The model under review builds one solid part; all positions refer to its coordinate system, in mm. Face numbers are marked on the shaded views. A direction names the side the tool comes from. Give positions to 0.01 mm unless a question says otherwise; leave off trailing zeros. Loops run counter-clockwise (first coordinate to the right, second up) from the corner with the lowest first, then second, coordinate; pieces in that order, holes last. Notation, with made-up numbers: M 76.5,43.5 L 130.5,43.5 A22 ccw 130.5,80.5 Z; hole C -12,24.25 d6. An arc over 180 degrees is marked long. Put each result on its own line as item: value. Start each with the question number.
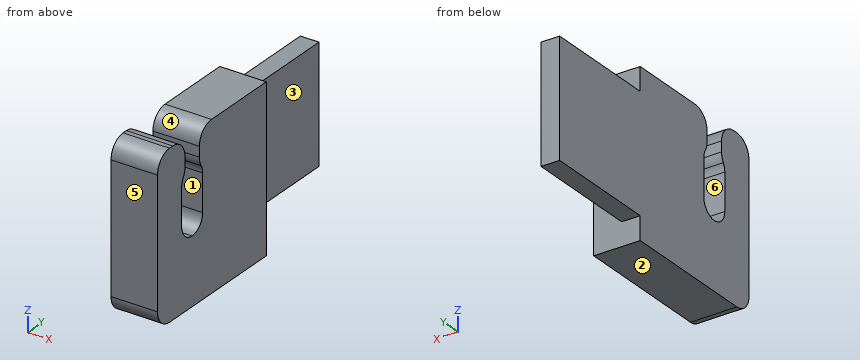
```python
from build123d import *

# Parameters (mm, degrees)
SKETCH1_W           = 10
SKETCH1_H           = 10
BOSS_EXTRUDE1_DEPTH = 1.6
BOSS_EXTRUDE2_DEPTH = 10
SKETCH3_W           = 4
SKETCH3_H           = 2
BOSS_EXTRUDE3_DEPTH = 2
SKETCH4_W           = 4
SKETCH4_H           = 2
BOSS_EXTRUDE4_DEPTH = 2
BOSS_EXTRUDE5_DEPTH = 4
FILLET1_R           = 1.5


with BuildPart() as part:
    # Sketch1 → Boss-Extrude1 (new body)
    with BuildSketch(Plane(origin=(0, 0, 0), x_dir=(0, 0, -1), z_dir=(1, 0, 0))):
        with Locations((5, -5)):
            Rectangle(SKETCH1_W, SKETCH1_H)
    extrude(amount=BOSS_EXTRUDE1_DEPTH)

    # Sketch2 → Boss-Extrude2 (add)
    with BuildSketch(Plane.XY):
        Polygon((1.2, -12), (0, -12), (0, -10), (1.6, -10), (4, -10), (4, -12), (2.8, -12), align=None)
    extrude(amount=-BOSS_EXTRUDE2_DEPTH)

    # Sketch3 → Boss-Extrude3 (add)
    with BuildSketch(Plane.XY):
        with Locations((2, -11)):
            Rectangle(SKETCH3_W, SKETCH3_H)
    extrude(amount=BOSS_EXTRUDE3_DEPTH)

    # Sketch4 → Boss-Extrude4 (add)
    with BuildSketch(Plane(origin=(0, 0, -10), x_dir=(-1, 0, 0), z_dir=(0, 0, -1))):
        with Locations((-2, -11)):
            Rectangle(SKETCH4_W, SKETCH4_H)
    extrude(amount=BOSS_EXTRUDE4_DEPTH)

    # Sketch5 → Boss-Extrude5 (add)
    with BuildSketch(Plane(origin=(4, 0, 0), x_dir=(0, 0, -1), z_dir=(1, 0, 0))):
        with BuildLine():
            Line((12, -12), (-2, -12))
            Line((-2, -12), (-2, -16.665516671))
            Line((-2, -16.665516671), (-2, -18.3))
            Line((-2, -18.3), (0.880666042, -18.3))
            ThreePointArc((0.880666042, -18.3), (1.308847242, -18.004173926), (1.818749194, -17.9))
            Line((1.818749194, -17.9), (5, -17.9))
            ThreePointArc((5, -17.9), (5.919238816, -18.280761184), (6.3, -19.2))
            ThreePointArc((6.3, -19.2), (5.919238816, -20.119238816), (5, -20.5))
            Line((5, -20.5), (1.818749194, -20.5))
            ThreePointArc((1.818749194, -20.5), (1.308847242, -20.395826074), (0.880666042, -20.1))
            Line((0.880666042, -20.1), (-2, -20.1))
            Line((-2, -20.1), (-2, -22))
            ThreePointArc((-2, -22), (-1.560660172, -23.060660172), (-0.5, -23.5))
            Line((-0.5, -23.5), (10.5, -23.5))
            ThreePointArc((10.5, -23.5), (11.560660172, -23.060660172), (12, -22))
            Line((12, -22), (12, -12))
        make_face()
    extrude(amount=-BOSS_EXTRUDE5_DEPTH)

    # Fillet1
    fillet1_edges = [part.edges().sort_by_distance(p)[0] for p in [
        (2, -18.3, -0.880666042),
        (2, -18.3, 2),
        (2, -20.1, 2),
        (2, -20.1, -0.880666042),
    ]]
    fillet(fillet1_edges, radius=FILLET1_R)


solid = part.part
```
Item 1: Tool access review of the marked faces 1, 2 and 3: name each direction out of +Z, -Z, +X, -X, +Y, -Y from which nothing blocks a thin tool from reaching the whole face with its end or side.
Item 2: To check wall thickness, follow L1, parallel to Y at x = 3.4, z = -3.25; L2, parallel to Y at x = 1.85, z = 0; L3, parallel to X at y = -3.5, z = -3.5. State the ranges of each line that lie inside material, in increasing order. Write a range as [from, to].
Item 3: Draft analysis for pull direction Z (two halves, no side actions). For the marked faces 4, 5 and 6, state which applies: +Z half, -Z half, draft (parallel to the pull), parting line (faces both ways), or undercut.
Item 4: Consider section A-A, the plane z = -0.75. Write out the cut boundary in (x, y).
Item 5: Consider section D-D, the plane y = -1.25. Write out the cut boundary in (x, z).
Item 6: Consider section C-C, the plane z = -8.5. Write out the cut boundary in (x, y).
Item 7: Consider section B-B, the plane x = 0.85. Write out the cut boundary in (y, z).
Item 8: Clearance check with flat-ended pins moving along their axes: pin 1 Ø1.5 at (x, y) = (1.5, -5) entering from +Z; pin 2 Ø8 at (y, z) = (-3.5, -5.5) entering from +X; pin 3 Ø1.2 at (x, z) = (1, -2.5) entering from +Y; pin 4 Ø1.6 at (x, z) = (2.5, -3.5) entering from +Y. State where each tip first meets the part, or that it passes through.
Report:
1. face 1: +X, -X
1. face 2: -Z, +X, -X, +Y, -Y
1. face 3: +Z, -Z, +X, +Y
2. L1: [-23.5, -20.5], [-17.9, -10]
2. L2: [-23.5, -20.1], [-18.3, -10]
2. L3: [0, 1.6]
3. face 4: +Z half
3. face 5: draft
3. face 6: undercut
4. outline: M 0,-23.5 L 4,-23.5 L 4,-20.15 L 0,-20.15 Z; M 0,-18.25 L 4,-18.25 L 4,-10 L 1.6,-10 L 1.6,0 L 0,0 Z
5. outline: M 0,-10 L 1.6,-10 L 1.6,0 L 0,0 Z
6. outline: M 0,-23.5 L 4,-23.5 L 4,-10 L 1.6,-10 L 1.6,0 L 0,0 Z
7. outline: M -23.5,-10.5 A1.5 ccw -22,-12 L -10,-12 L -10,-10 L 0,-10 L 0,0 L -10,0 L -10,2 L -16.8,2 A1.5 ccw -18.3,0.5 L -18.3,-0.38 A1.5 ccw -18.09,-1.15 A1.3 cw -17.9,-1.82 L -17.9,-5 A1.3 cw -20.5,-5 L -20.5,-1.82 A1.3 cw -20.31,-1.15 A1.5 ccw -20.1,-0.38 L -20.1,0.5 A1.5 ccw -21.6,2 L -22,2 A1.5 ccw -23.5,0.5 Z
8. pin 1: z = 0
8. pin 2: x = 1.6
8. pin 3: y = 0
8. pin 4: y = -10
